from build123d import *

# Parameters (mm, degrees)
SKETCH2_R           = 50
BOSS_EXTRUDE1_DEPTH = 100
SKETCH3_W           = 200
SKETCH3_H           = 100
BOSS_EXTRUDE2_DEPTH = 50
CUT_EXTRUDE1_DEPTH  = 255.95097568
SKETCH5_R           = 5
BOSS_EXTRUDE3_DEPTH = 10


with BuildPart() as part:
    # Sketch2 → Boss-Extrude1 (new body)
    with BuildSketch(Plane(origin=(0, 0, 0), x_dir=(1, 0, 0), z_dir=(0, 1, 0))):
        with Locations(Location((0, 0, 0), (0, 0, 270))):
            Circle(SKETCH2_R)
    extrude(amount=BOSS_EXTRUDE1_DEPTH)

    # Sketch3 → Boss-Extrude2 (add)
    with BuildSketch(Plane(origin=(0, 100, 0), x_dir=(1, 0, 0), z_dir=(0, 1, 0))):
        Rectangle(SKETCH3_W, SKETCH3_H)
    extrude(amount=BOSS_EXTRUDE2_DEPTH)

    # Sketch4 → Cut-Extrude1 (cut, through all)
    with BuildSketch(Plane(origin=(100, 0, 0), x_dir=(0, 0, -1), z_dir=(1, 0, 0))):
        Polygon((-35, 150), (-35, 135), (-40, 135), (-40, 125), (-10, 125), (-10, 135), (-15, 135), (-15, 150), align=None)
        Polygon((40, 135), (40, 125), (10, 125), (10, 135), (15, 135), (15, 150), (35, 150), (35, 135), align=None)
    extrude(amount=-CUT_EXTRUDE1_DEPTH, mode=Mode.SUBTRACT)

    # Sketch5 → Boss-Extrude3 (add)
    with BuildSketch(Plane(origin=(0, 150, 0), x_dir=(1, 0, 0), z_dir=(0, 1, 0))):
        with Locations(Location((0, 0, 0), (0, 0, 270))):
            Circle(SKETCH5_R)
    extrude(amount=BOSS_EXTRUDE3_DEPTH)


solid = part.part
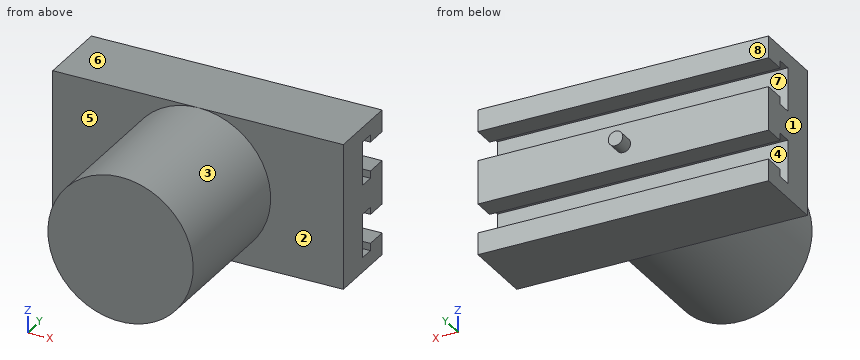
Could you check a few things on this model? Use its own coordinates, in mm. Face numbers are marked on the shaded views. A direction names the side the tool comes from. Give positions to 0.01 mm unless a question says otherwise; leave off trailing zeros. Order: outer loops, then holes, each group sorted by start corner. A loop starts at its lowest first (then second) coordinate and runs counter-clockwise, first axis right, second up.
1. Suppose I cut it at A-A (y = 145). Write out the boundary of the cut face in (x, z), plus the area to 3 significant figures.
Answers below:
outline: (-100, -50) - (100, -50) - (100, -35) - (-100, -35) - close; (-100, -15) - (100, -15) - (100, 15) - (-100, 15) - close; (-100, 35) - (100, 35) - (100, 50) - (-100, 50) - close
area: 12,000 mm2
2. Suppose I cut it at B-B (z = 0). Write out the boundary of the cut face in (x, y).
Answers below:
outline: (-100, 100) - (-50, 100) - (-50, 0) - (50, 0) - (50, 100) - (100, 100) - (100, 150) - (5, 150) - (5, 160) - (-5, 160) - (-5, 150) - (-100, 150) - close
3. Which directions (+Z, -Z, +X, -X, +Y, -Y) give clear straight access to the entire face, cutting with the end or side of a thin tool? Please do the marked faces 1, 2, 3 and 4.
Answers below:
face 1: +Z, -Z, -X, +Y, -Y
face 2: +X, -Y
face 3: -Y
face 4: +X, -X
4. For pin 1 (1.5 mm diameter, centred on x = 76, z = 35, fed in from -Y); pin 2 (1.5 mm diameter, centred on x = -22, z = -37, fed in from -Y); pin 3 (9 mm diameter, centred on x = -7, z = 23, fed in from +Y); pin 4 (7.5 mm diameter, centred on x = 33.5, z = -43.5, fed in from +Y), each with a flat end and sliding along its axis, tell me the tip position at first contact or that it passes through.
Answers below:
pin 1: stops at y = 100
pin 2: stops at y = 0
pin 3: stops at y = 125
pin 4: stops at y = 150
5. Suppose I cut it at D-D (y = 37). Write out the boundary of the cut face in (x, z), plus the area to 3 significant figures.
Answers below:
outline: circle Ø100 at (0, 0)
area: 7,850 mm2
6. Thinking about a two-plate mould opening in Y: for the marked faces 5, 6, 7 and 8, which applies, +Y half, -Y half, draft (parallel to the pull), parting line (faces both ways), or undercut?
Answers below:
face 5: -Y half
face 6: draft
face 7: undercut
face 8: +Y half
7. Suppose I cut it at C-C (x = 45.5). Write out the boundary of the cut face in (y, z).
Answers below:
outline: (0, -20.73) - (100, -20.73) - (100, -50) - (150, -50) - (150, -35) - (135, -35) - (135, -40) - (125, -40) - (125, -10) - (135, -10) - (135, -15) - (150, -15) - (150, 15) - (135, 15) - (135, 10) - (125, 10) - (125, 40) - (135, 40) - (135, 35) - (150, 35) - (150, 50) - (100, 50) - (100, 20.73) - (0, 20.73) - close
8. I need wall thicknesses on L1, parallel to Z at x = 73.5, y = 145.5; L2, parallel to Y at x = 9, z = 3.5; L3, parallel to Y at x = 35.5, z = 14.5. Which ranges of each line are inside material? Lowest first, please.
Answers below:
L1: z = -50 to -35, -15 to 15, 35 to 50
L2: y = 0 to 150
L3: y = 0 to 125, 135 to 150
